Part model, mm, in its own coordinate system. A direction names the side the tool comes from. Coordinates: 2 decimals unless noted, no trailing zeros. Loops run counter-clockwise (first coordinate to the right, second up) from the corner with the lowest first, then second, coordinate; pieces in that order, holes last. Notation, with made-up numbers: (19, 34.25) - (52, 34.25) arc R4 cw to (52, 41.25) - close; hole circle Ø3 at (-11, -31.75). An arc over 180 degrees is marked (long way). Use a Markdown table: item, result. Add a question column.
1. Drop flat-ended pins along their axis: pin 1 (1.5 mm diameter, centred on x = 42.5, y = 37.5, fed in from +Z); pin 2 (0.9 mm diameter, centred on x = 41.5, z = 282, fed in from -Y); pin 3 (0.9 mm diameter, centred on x = 42, y = -1.5, fed in from +Z). Give the stop position or say it passes through.
2. Band-saw the part on B-B, the plane y = 26. Give the cut face in (x, z), plus the area to 3 significant figures.
3. Band-saw the part on C-C, the plane y = 14. Give the cut face in (x, z), plus the area to 3 significant figures.
4. 3-axis set-ups, long thin cutter, end or side, ignore diameter. For faces 4 (the flat face through (41, 34, 140)), 5 (the flat face through (41, -2, 156)), 6 (the flat face through (41, 75, 222)), 7 (the flat face through (41, 8, 278)), 8 (the flat face through (42, 37, 145)): which of +Z, -Z, +X, -X, +Y, -Y reach the whole face in a straight line?
5. Band-saw the part on D-D, the plane z = 292. Give the cut face in (x, y).
6. Pull direction Y, two halves, no side cores. Call faces 1 (the flat face through (41, 31, 317)), 2 (the cylindrical face through (41.52, 59.74, 148.58)), 3 (the flat face through (40, 43, 231)): pulls with the +Y half, pulls with the -Y half, needs draft (parallel to the pull), parting line crosses it, or undercut.
7. Band-saw the part on A-A, the plane z = 150. Give the cut face in (x, y), plus the area to 3 significant figures.
8. Wall check: probe 1 along Z at (x, y) = (41.45, 70); probe 2 along Y at (x, z) = (42.1, 150); probe 3 along Z at (x, y) = (41.45, 59). Give the ranges that are in metal, low to high. Write a range as [from, to].
from build123d import *

# Parameters (mm, degrees)
SKETCH_R        = 1.6
PAD_DEPTH       = 3
CHAMFER_SIZE    = 1
POCKET014_DEPTH = 3.001
CHAMFER059_SIZE = 1
SKETCH159_R     = 1.6
POCKET015_DEPTH = 43.001
SKETCH188_W     = 37.119205
SKETCH188_H     = 78.955215
SKETCH188_W_2   = 7
SKETCH188_H_2   = 30
PAD099_DEPTH    = 3
SKETCH189_R     = 1.6
POCKET032_DEPTH = 3.001
SKETCH190_W     = 3
SKETCH190_H     = 55
PAD100_DEPTH    = 3
CHAMFER065_SIZE = 1
FILLET066_R     = 2


with BuildPart() as part:
    # Sketch → Pad (new body)
    with BuildSketch(Plane.YZ.offset(40)):
        with BuildLine():
            Line((8, 320), (31, 320))
            Line((31, 320), (31, 315))
            ThreePointArc((31, 315), (33.343146, 309.343146), (39, 307))
            Line((75, 307), (39, 307))
            Line((75, 140), (75, 307))
            Line((-5, 140), (75, 140))
            Line((-5, 156), (-5, 140))
            Line((-5, 156), (0, 156))
            ThreePointArc((0, 156), (4, 160), (0, 164))
            Line((0, 164), (-5, 164))
            Line((-5, 180), (-5, 164))
            Line((8, 180), (-5, 180))
            Line((8, 320), (8, 180))
        make_face()
        with Locations((19.5, 315)):
            Circle(SKETCH_R, mode=Mode.SUBTRACT)
        with Locations((70, 292)):
            Circle(SKETCH_R, mode=Mode.SUBTRACT)
        with Locations((70, 155)):
            Circle(SKETCH_R, mode=Mode.SUBTRACT)
    extrude(amount=PAD_DEPTH)

    # Chamfer
    chamfer_edges = [part.edges().sort_by_distance(p)[0] for p in [
        (41.5, -5, 180),
        (41.5, 8, 180),
        (41.5, -5, 164),
        (41.5, -5, 156),
        (41.5, -5, 140),
        (41.5, 75, 140),
        (41.5, 75, 307),
        (41.5, 8, 320),
        (41.5, 31, 320),
    ]]
    chamfer(chamfer_edges, length=CHAMFER_SIZE)

    # Sketch158 (on Face5 of Chamfer) → Pocket014 (cut, through all)
    with BuildSketch(Plane.YZ.offset(43)):
        with BuildLine():
            ThreePointArc((54, 140), (56.5, 137.5), (59, 140))
            Line((59, 140), (59, 160))
            ThreePointArc((59, 160), (56.5, 162.5), (54, 160))
            Line((54, 160), (54, 140))
        make_face()
    extrude(amount=-POCKET014_DEPTH, mode=Mode.SUBTRACT)

    # Chamfer059
    chamfer059_edges = [part.edges().sort_by_distance(p)[0] for p in [
        (41.5, 54, 140),
        (41.5, 59, 140),
    ]]
    chamfer(chamfer059_edges, length=CHAMFER059_SIZE)

    # Sketch159 → Pocket015 (cut, through all)
    with BuildSketch(Plane.YZ):
        with Locations((18, 260)):
            Circle(SKETCH159_R)
        with Locations((35.78, 260)):
            Circle(SKETCH159_R)
        with Locations((18, 204.76)):
            Circle(SKETCH159_R)
        with Locations((35.78, 204.76)):
            Circle(SKETCH159_R)
    extrude(amount=POCKET015_DEPTH, mode=Mode.SUBTRACT)

    # Sketch188 (on Face37 of Clone004) → Pad099 (new body)
    with BuildSketch(Plane.YZ.offset(43)):
        with Locations((30.900274, 230.820335)):
            Rectangle(SKETCH188_W, SKETCH188_H)
        with Locations((56.5, 155)):
            Rectangle(SKETCH188_W_2, SKETCH188_H_2)
    extrude(amount=-PAD099_DEPTH)

    # Sketch189 (on Face27 of Pad099) → Pocket032 (cut, through all)
    with BuildSketch(Plane.YZ.offset(43)):
        with Locations((14, 260)):
            Circle(SKETCH189_R)
        with Locations((59, 260)):
            Circle(SKETCH189_R)
        with Locations((59, 150)):
            Circle(SKETCH189_R)
        with Locations((14, 150)):
            Circle(SKETCH189_R)
        Polygon((10, 225), (52, 225), (52, 191), (64, 191), (64, 160), (55, 160), (55, 145), (18, 145), (18, 160), (10, 160), align=None)
    extrude(amount=-POCKET032_DEPTH, mode=Mode.SUBTRACT)

    # Sketch190 (on Face5 of Pocket032) → Pad100 (join)
    with BuildSketch(Plane.YZ.offset(43)):
        with Locations((6.5, 207.5)):
            Rectangle(SKETCH190_W, SKETCH190_H)
    extrude(amount=-PAD100_DEPTH)

    # Chamfer065
    chamfer065_edges = [part.edges().sort_by_distance(p)[0] for p in [
        (41.5, 5, 180),
        (41.5, 5, 235),
        (41.5, 8, 235),
    ]]
    chamfer(chamfer065_edges, length=CHAMFER065_SIZE)

    # Fillet066
    fillet066_edges = [part.edges().sort_by_distance(p)[0] for p in [
        (41.5, 18, 160),
        (41.5, 55, 160),
        (41.5, 52, 191),
        (41.5, 64, 160),
        (41.5, 64, 191),
        (41.5, 52, 225),
        (41.5, 10, 225),
        (41.5, 10, 160),
        (41.5, 55, 145),
        (41.5, 18, 145),
    ]]
    fillet(fillet066_edges, radius=FILLET066_R)


solid = part.part
Geometry check:
| question | item | result |
|---|---|---|
| 1 | pin 1 | stops at z = 307.32 |
| 1 | pin 2 | stops at y = 8 |
| 1 | pin 3 | stops at z = 180 |
| 2 | outline | (40, 140) - (43, 140) - (43, 145) - (40, 145) - close; (40, 225) - (43, 225) - (43, 320) - (40, 320) - close |
| 2 | area | 300 mm^2 |
| 3 | outline | (40, 140) - (43, 140) - (43, 148.4) - (40, 148.4) - close; (40, 151.6) - (43, 151.6) - (43, 160) - (40, 160) - close; (40, 225) - (43, 225) - (43, 258.4) - (40, 258.4) - close; (40, 261.6) - (43, 261.6) - (43, 320) - (40, 320) - close |
| 3 | area | 326 mm^2 |
| 4 | face 4 | -Z, +X, -X, +Y, -Y |
| 4 | face 5 | +X, -X, -Y |
| 4 | face 6 | +Z, -Z, +X, -X, +Y |
| 4 | face 7 | +Z, +X, -X, -Y |
| 4 | face 8 | +X, -X |
| 5 | outline | (40, 8) - (43, 8) - (43, 68.4) - (40, 68.4) - close; (40, 71.6) - (43, 71.6) - (43, 75) - (40, 75) - close |
| 6 | face 1 | pulls with the +Y half |
| 6 | face 2 | undercut |
| 6 | face 3 | needs draft |
| 7 | outline | (40, -5) - (43, -5) - (43, 12.4) - (40, 12.4) - close; (40, 15.6) - (43, 15.6) - (43, 18) - (40, 18) - close; (40, 55) - (43, 55) - (43, 57.4) - (40, 57.4) - close; (40, 60.6) - (43, 60.6) - (43, 75) - (40, 75) - close |
| 7 | area | 110 mm^2 |
| 8 | probe 1 | z = [140, 153.4], [156.6, 290.4], [293.6, 307] |
| 8 | probe 2 | y = [-5, 12.4], [15.6, 18], [55, 57.4], [60.6, 75] |
| 8 | probe 3 | z = [140, 148.4], [151.6, 160], [191, 258.4], [261.6, 307] |
